Source: CAD feature listing. Evaluate the final solid. Frame: model axes, mm. A direction names the side the tool comes from. Coordinates: 2 decimals unless noted, no trailing zeros. Write each loop counter-clockwise with the first axis right and the second up, starting at its lowest first coordinate (ties: lowest second). Pieces come first, ordered by that corner, then holes. Notation, with made-up numbers: (-6.5, 35) - (6.5, 35) arc R30 cw to (6.5, 72) - close; hole circle Ø11 at (55.25, -35). An arc over 180 degrees is marked (long way). One line per question, with ' | ' between items.
Autodesk Inventor part; units mm, degrees
ref_plane "YZ Plane" through (0, 0, 0) normal (1, 0, 0) x (0, 1, 0)
ref_plane "XZ Plane" through (0, 0, 0) normal (0, 1, 0) x (-1, 0, 0)
ref_plane "XY Plane" through (0, 0, 0) normal (0, 0, 1) x (1, 0, 0)
sketch "Sketch1" plane through (0, 0, 0) normal (0, 0, 1) x (1, 0, 0)
  line L0 (-22.225, 0) -> (22.225, 0)
  line L1 (0, -22.225) -> (0, 22.225)
  circle A0 centre (0, 0) radius 15.875
  circle A1 centre (0, 0) radius 6.35
  dimension "d0" = 12.7
  dimension "d1" = 31.75
extrude "Base" add sketch "Sketch1" along normal mid plane 7.9375 contours A1 L1 A0 L0 | L0 A0 L1 A1 | A1 L0 A0 L1 | L1 A0 L0 A1
sketch "Sketch2" plane through (0, 0, 3.9688) normal (0, 0, 1) x (1, 0, 0)
  circle A0 centre (0, 0) radius 15.875
  circle A1 centre (0, 0) radius 14.2875
  dimension "d4" = 28.575
extrude "Flange Cutaway" cut sketch "Sketch2" against normal blind 6.3627
sketch "Sketch3" plane through (0, 0, 3.9688) normal (0, 0, 1) x (1, 0, 0)
  circle A0 centre (0, 0) radius 14.2875
  circle A1 centre (0, 0) radius 6.35
  circle A2 centre (0, 0) radius 7.9375
  circle A3 centre (0, 0) radius 11.9062
  dimension "d7" = 1.5875
  dimension "d8" = 2.3813
extrude "Cutaway" cut sketch "Sketch3" against normal blind 0.3969 contours A3
mirror "Mirror1" about plane through (0, 0, 0) normal (0, 0, 1) of "Cutaway"
properties part number "bearing_1.125OD" material "Steel"
Item 1: Ray query, line 1 along X through (y, z) = (0, -3) (3 decimals); line 2 along Z through (x, y) = (8, 13); line 3 along Y through (x, z) = (5, -3.5). Return the intervals inside material, ascending. Write a range as [from, to].
Check sheet entries:
line 1: [-15.875, -6.35], [6.35, 15.875] | line 2: [-3.97, -2.39] | line 3: [-15.07, -3.91], [3.91, 15.07]
Item 2: Cut plane C-C on y = 13. Return loops of the section in (x, z).
Check sheet entries:
outline: (-9.11, -3.97) - (9.11, -3.97) - (9.11, -2.39) - (5.93, -2.39) - (5.93, 3.97) - (-5.93, 3.97) - (-5.93, -2.39) - (-9.11, -2.39) - close
Item 3: Pin query (flat end, axial travel): pin 1 Ø1.5 at (y, z) = (3.5, 2.5) entering from +X; pin 2 Ø3 at (x, z) = (8.5, 2) entering from +Y. Return the tip coordinate at first contact, or that it passes through.
Check sheet entries:
pin 1: x = 14.02 | pin 2: y = 12.46
Item 4: Cut plane D-D on z = -3. Return loops of the section in (x, y) (3 decimals).
Check sheet entries:
outline: circle Ø31.75 at (0, 0); hole circle Ø12.7 at (0, 0)
Item 5: Access query for faces 1 (the face through (-1.72, 7.75, -3.77)), 2 (the face through (-1.38, 6.2, -0.06)), 3 (the face through (-1.72, -7.75, 3.77)). Directions: +Z, -Z, +X, -X, +Y, -Y. A direction counts if a zero-diameter tool reaches every point of the face in a straight line with its end or side. Return the directions, or none.
Check sheet entries:
face 1: -Z | face 2: +Z, -Z | face 3: +Z
Item 6: Mould query, pull axis Y, two halves, no side actions, for faces 4 (the face through (-14.274, 0.628, 0.832)), 5 (the face through (-2.581, -11.623, 3.773)), 6 (the face through (-2, -8, -3.572)), 7 (the face through (-11.83, 8.31, -2.394)). Classes: pulls with the +Y half, pulls with the -Y half, needs draft (parallel to the pull), parting line crosses it, or undercut.
Check sheet entries:
face 4: parting line crosses it | face 5: undercut | face 6: undercut | face 7: needs draft
